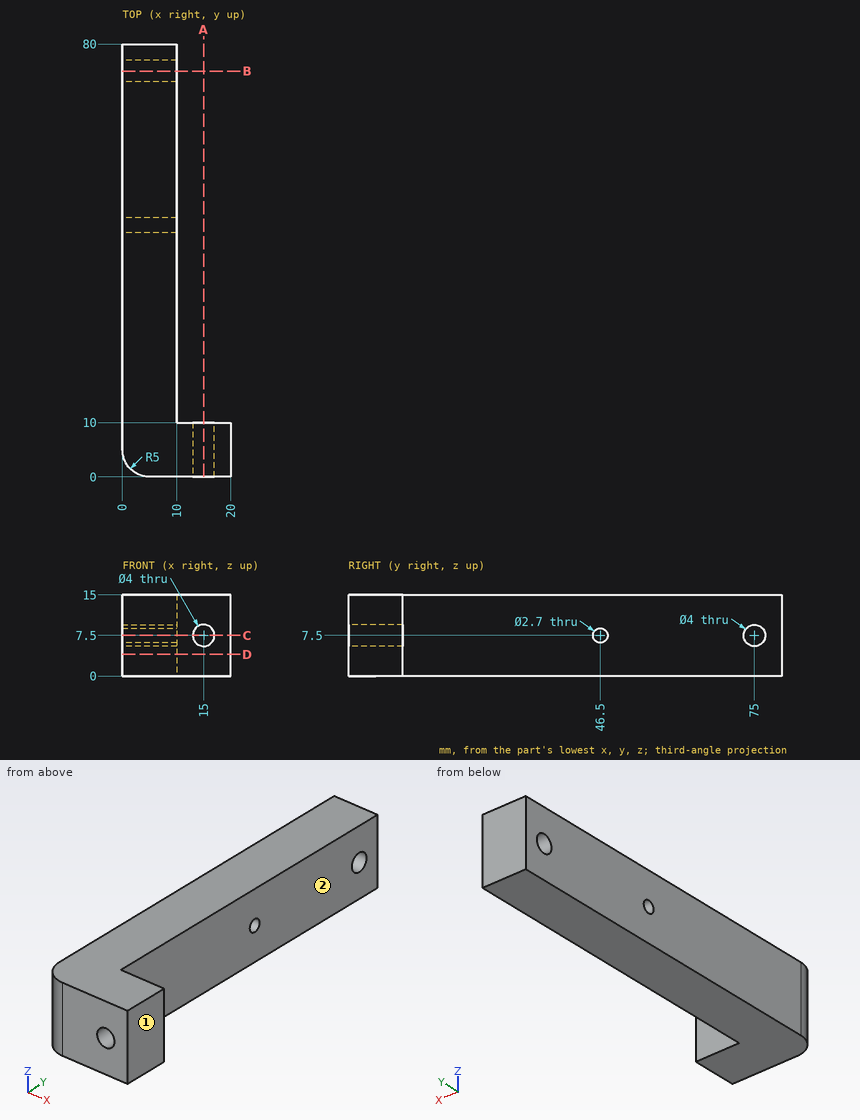
Input: dimensioned drawing with shaded views. Units: mm. Origin: part minimum x, y, z. A direction names the side the tool comes from. Give positions to 0.01 mm unless a question says otherwise; leave off trailing zeros. Loops run counter-clockwise (first coordinate to the right, second up) from the corner with the lowest first, then second, coordinate; pieces in that order, holes last. Notation, with made-up numbers: (-25, 58) - (-16, 58) arc R23 cw to (-16, 92) - close; hole circle Ø3 at (38, -6). An arc over 180 degrees is marked (long way). Answer as CSV lines item,"result". Start each with the question number.
(1) Section query C-C (z = 7.5). Output: boundary loops of the cut face in (x, y), and give its area (3 significant figures).
(2) Section query D-D (z = 4). Output: boundary loops of the cut face in (x, y), and give its area (3 significant figures).
(3) Ray query, line 1 along Y through (x, z) = (6, 7.5); line 2 along Z through (x, y) = (6.75, 46.5); line 3 along Z through (x, y) = (15, 7.25). Return the intervals inside material, ascending. Write a range as [from, to].
(4) Section query A-A (x = 15). Output: boundary loops of the cut face in (y, z).
(5) Pin query (flat end, axial travel): P1, Ø5, axis at x = 2, z = 12.5, coming from the -Y side; P2, Ø4.5, axis at y = 47.5, z = 6.5, coming from the +X side; P3, Ø2, axis at x = 16.5, z = 8.5, coming from the +Y side. Return the tip coordinate at first contact, or that it passes through.
(6) Reachability of the marked faces 1 and 2 from +Z, -Z, +X, -X, +Y, -Y: full face, straight path, thin tool, end or side. Return the list, or none.
Worked answers:
1,outline,"(0, 5) arc R5 ccw to (5, 0) - (13, 0) - (13, 10) - (10, 10) - (10, 45.15) - (0, 45.15) - close; (0, 47.85) - (10, 47.85) - (10, 73) - (0, 73) - close; (0, 77) - (10, 77) - (10, 80) - (0, 80) - close; (17, 0) - (20, 0) - (20, 10) - (17, 10) - close"
1,area,"788 mm^2"
2,outline,"(0, 5) arc R5 ccw to (5, 0) - (20, 0) - (20, 10) - (10, 10) - (10, 80) - (0, 80) - close"
2,area,"895 mm^2"
3,line 1,"y = [0, 45.15], [47.85, 73], [77, 80]"
3,line 2,"z = [0, 6.15], [8.85, 15]"
3,line 3,"z = [0, 5.5], [9.5, 15]"
4,outline,"(0, 0) - (10, 0) - (10, 5.5) - (0, 5.5) - close; (0, 9.5) - (10, 9.5) - (10, 15) - (0, 15) - close"
5,P1,"stops at y = 0.03"
5,P2,"stops at x = 10"
5,P3,"stops at y = 10"
6,face 1,"+Z, -Z, +X, +Y, -Y"
6,face 2,"+Z, -Z, +X, +Y"
